Build history of the part. All positions in model axes, mm. A direction names the side the tool comes from. Coordinates: 2 decimals unless noted, no trailing zeros. Order: outer loops, then holes, each group sorted by start corner. A loop starts at its lowest first (then second) coordinate and runs counter-clockwise, first axis right, second up. Notation, with made-up numbers: (58.25, -25.5) - (95.25, -25.5) arc R12 ccw to (95.25, -18.5) - close; hole circle Ø11 at (30.25, -37). An arc over 180 degrees is marked (long way). Return JSON: item names as keys, results as strings.
from build123d import *

# Parameters (mm, degrees)
ESBO_O1_W                                         = 40
ESBO_O1_H                                         = 38
RESSALTO_EXTRUS_O1_DEPTH                          = 8
ESBO_O2_R                                         = 11
CORTE_EXTRUS_O1_DEPTH                             = 7
FURO_ROSCADO_PARA_CONDU_TE_DE_M3X0_51_D           = 3.15
FURO_ROSCADO_PARA_CONDU_TE_DE_M3X0_51_DEPTH       = 10
FURO_ROSCADO_PARA_CONDU_TE_DE_M3X0_51_CSINK_D     = 3.766
FURO_ROSCADO_PARA_CONDU_TE_DE_M3X0_51_CSINK_ANGLE = 90
FURO_ROSCADO_PARA_CONDU_TE_DE_M3X0_51_TIP         = 0.946355475


with BuildPart() as part:
    # Esboço1 → Ressalto-extrusão1 (new body)
    with BuildSketch(Plane.XY):
        Rectangle(ESBO_O1_W, ESBO_O1_H)
    extrude(amount=RESSALTO_EXTRUS_O1_DEPTH)

    # Esboço2 → Corte-extrusão1 (cut)
    with BuildSketch(Plane.XY.offset(8)):
        with Locations((0, 4.5)):
            Circle(ESBO_O2_R)
    extrude(amount=-CORTE_EXTRUS_O1_DEPTH, mode=Mode.SUBTRACT)

    # Furo roscado para conduíte de M3x0.51
    with Locations(Plane(origin=(0, -19, 0), x_dir=(-1, 0, 0), z_dir=(0, -1, 0))):
        with Locations((-12, -4), (12, -4)):
            CounterSinkHole(FURO_ROSCADO_PARA_CONDU_TE_DE_M3X0_51_D / 2, FURO_ROSCADO_PARA_CONDU_TE_DE_M3X0_51_CSINK_D / 2, depth=FURO_ROSCADO_PARA_CONDU_TE_DE_M3X0_51_DEPTH, counter_sink_angle=FURO_ROSCADO_PARA_CONDU_TE_DE_M3X0_51_CSINK_ANGLE)
            with Locations((0, 0, -(FURO_ROSCADO_PARA_CONDU_TE_DE_M3X0_51_DEPTH + FURO_ROSCADO_PARA_CONDU_TE_DE_M3X0_51_TIP / 2))):  # 118° drill point
                Cone(0, FURO_ROSCADO_PARA_CONDU_TE_DE_M3X0_51_D / 2, FURO_ROSCADO_PARA_CONDU_TE_DE_M3X0_51_TIP, mode=Mode.SUBTRACT)


solid = part.part
1. Drop flat-ended pins along their axis: pin 1 (20 mm diameter, centred on x = 0, y = 4.5, fed in from +Z); pin 2 (4 mm diameter, centred on x = 12, z = 4, fed in from -Y). Give the stop position or say it passes through.
Check values:
{"pin 1": "z = 1", "pin 2": "y = -19"}
2. Cut at D-D on y = 4.5. Give the cut face in (x, z), plus the area to 3 significant figures.
Check values:
{"outline": "(-20, 0) - (20, 0) - (20, 8) - (11, 8) - (11, 1) - (-11, 1) - (-11, 8) - (-20, 8) - close", "area": "166 mm²"}
3. Cut at C-C on x = 0. Give the cut face in (y, z).
Check values:
{"outline": "(-19, 0) - (19, 0) - (19, 8) - (15.5, 8) - (15.5, 1) - (-6.5, 1) - (-6.5, 8) - (-19, 8) - close"}
4. Probe L1, parallel to X at y = -15.5, z = 4 (3 decimals); L2, parallel to Y at x = 0, z = 3.75; L3, parallel to Z at x = 12, y = -12.5 (3 decimals). List the from-to ranges inside material, lowest first.
Check values:
{"L1": "-20 to -13.575, -10.425 to 10.425, 13.575 to 20", "L2": "-19 to -6.5, 15.5 to 19", "L3": "0 to 2.425, 5.575 to 8"}
5. Cut at B-B on z = 6.5. Give the cut face in (x, y).
Check values:
{"outline": "(-20, -19) - (20, -19) - (20, 19) - (-20, 19) - close; hole circle Ø22 at (0, 4.5)"}
6. Mould opens along Y. For faces 3 (the flat face through (0, -8, 8)), 4 (the cylindrical face through (-2.38, -6.24, 4.55)), 5 (the conical face through (12.273, -8.218, 3.988)), 6 (the flat face through (0, 5, 1)) say: pulls with the +Y half, pulls with the -Y half, needs draft (parallel to the pull), parting line crosses it, or undercut.
Check values:
{"face 3": "needs draft", "face 4": "undercut", "face 5": "pulls with the -Y half", "face 6": "undercut"}
7. Tool access for faces 1 (the cylindrical face through (11.79, -13.78, 2.44)), 2 (the flat face through (20, 0, 4)): list every direction of +Z, -Z, +X, -X, +Y, -Y with a clear straight run to the whole face (end or side of a thin tool).
Check values:
{"face 1": "-Y", "face 2": "+Z, -Z, +X, +Y, -Y"}
8. Cut at A-A on y = -16. Give the cut face in (x, z) (3 decimals), plus the area to 3 significant figures.
Check values:
{"outline": "(-20, 0) - (20, 0) - (20, 8) - (-20, 8) - close; hole circle Ø3.15 at (-12, 4); hole circle Ø3.15 at (12, 4)", "area": "304 mm²"}
